Autodesk Inventor part; units mm, degrees
ref_plane "YZ Plane" through (0, 0, 0) normal (1, 0, 0) x (0, 1, 0)
ref_plane "XZ Plane" through (0, 0, 0) normal (0, 1, 0) x (-1, 0, 0)
ref_plane "XY Plane" through (0, 0, 0) normal (0, 0, 1) x (1, 0, 0)
sketch "Boceto1" plane through (0, 0, 0) normal (0, 1, 0) x (-1, 0, 0)
  line L0 (0, 0) -> (11, 0)
  line L1 (11, 0) -> (11, -11)
  line L2 (11, -11) -> (0, -11)
  line L3 (0, -11) -> (0, 0)
  dimension "d0" = 11
  dimension "d1" = 11
extrude "Extrusión1" add sketch "Boceto1" along normal blind 1.25
sketch "Boceto2" plane through (0, 1.25, 0) normal (0, 1, 0) x (1, 0, 0)
  line L0 (-11, 0) -> (0, 0)
  line L1 (-11, 11) -> (-11, 0)
  line L2 (0, 0) -> (-11, 11)
  line L3 (0, 0) -> (0, 11)
  line L4 (0, 11) -> (-11, 0)
  circle A0 centre (-5.5, 5.5) radius 5.5
  dimension "d4" = 11
extrude "Extrusión2" add sketch "Boceto2" along normal blind 6 contours A0 L4 L2 | A0 L2 L4 | L2 L4 A0 | A0 L4 L2
sketch "Boceto4" plane through (-5.5, 7.25, -5.5) normal (0, 1, 0) x (1, 0, 0)
  line L0 (0, 0) -> (-3, 0)
  line L1 (-3, 0) -> (-3, 1.5)
  line L2 (-3, 1.5) -> (-3, -1.5)
  line L3 (-3, -1.5) -> (-1.5, -1.5)
  line L4 (-1.5, -1.5) -> (-1.5, -3)
  line L5 (-1.5, -3) -> (1.5, -3)
  line L6 (1.5, -3) -> (1.5, -1.5)
  line L7 (1.5, -1.5) -> (3, -1.5)
  line L8 (3, -1.5) -> (3, 1.5)
  line L9 (3, 1.5) -> (1.5, 1.5)
  line L10 (1.5, 1.5) -> (1.5, 3)
  line L11 (1.5, 3) -> (-1.5, 3)
  line L12 (-1.5, 3) -> (-1.5, 1.5)
  line L13 (-3, 1.5) -> (-1.5, 1.5)
  line L14 (-1.5, 1.5) -> (-1.5, -1.5)
  line L15 (1.5, -1.5) -> (1.5, 1.5)
  line L16 (-1.5, 1.5) -> (1.5, 1.5)
  line L17 (1.5, -1.5) -> (-1.5, -1.5)
  point P0 (5.5, -5.5)
  dimension "d7" = 3
  dimension "d8" = 1.5
  dimension "d9" = 3
  dimension "d10" = 1.5
  dimension "d11" = 1.5
  dimension "d12" = 3
  dimension "d13" = 1.5
  dimension "d14" = 1.5
  dimension "d15" = 3
  dimension "d16" = 1.5
  dimension "d17" = 1.5
  dimension "d18" = 3
extrude "Extrusión3" cut sketch "Boceto4" against normal blind 5 contours L14 L16 L15 L17
sketch "Boceto8" plane through (-5.5, 7.25, -5.5) normal (0, 1, 0) x (1, 0, 0)
  circle A0 centre (0, 0) radius 2.75
  circle A1 centre (0, 0) radius 4.5
  point P0 (5.5, -5.5)
  dimension "d47" = 5.5
  dimension "d48" = 9
extrude "Extrusión6" cut sketch "Boceto8" against normal blind 2
fillet "Empalme4" radius 1 4 edges at (-7, 4.75, -7) (-4, 4.75, -7) (-4, 4.75, -4) (-7, 4.75, -4)
properties part number "Boton Base"
Verification items for the finished model (mm, model axes). A direction names the side the tool comes from. Round coordinates to 2 decimals unless told otherwise and drop trailing zeros. Order: outer loops, then holes, each group sorted by start corner. A loop starts at its lowest first (then second) coordinate and runs counter-clockwise, first axis right, second up. Notation, with made-up numbers: (40.5, 73.5) -> (95.5, 73.5) arc R27 ccw to (95.5, 103.5) -> close; hole circle Ø11 at (29.25, 76). An arc over 180 degrees is marked (long way). Put each result on its own line as item: value. Start each with the question number.
(1) Section check B-B (y = 3.5). Enter the section's corners in (x, z), then the cut area to 3 significant figures.
(2) Tool access check on faces 5 (the face through (-10, 1.25, -10)), 6 (the face through (-4.301, 4.715, -6.715)), 7 (the face through (-10, 1.25, -1)). Record the directions out of +Z, -Z, +X, -X, +Y, -Y that give a thin tool (end or side, any length) a straight path to the whole face; none if there is none.
(3) Section check D-D (x = -2.25). Enter the section's corners in (y, z), then the cut area to 3 significant figures.
(4) Section check A-A (y = 6). Enter the section's corners in (x, z).
(5) Depth check by flat-ended pin: pin 1 Ø2 at (x, y) = (-4.5, 4) entering from -Z; pin 2 Ø3 at (x, y) = (-2.5, 6.5) entering from -Z; pin 3 Ø1 at (y, z) = (3.5, -1.5) entering from -X. Enter the tip coordinate at first touch or a pass-through.
(6) Draft check along Z on faces 1 (the face through (0, 1, -6)), 2 (the face through (-6, 1, -11)), 3 (the face through (-6.69, 4.21, -10.87)), 4 (the face through (-4.23, 6.26, -3.06)). Enter one of: +Z half, -Z half, draft (parallel to the pull), parting line (faces both ways), or undercut.
(7) Material ranges on line 1 along X through (y, z) = (6.8, -5.5); line 2 along Z through (x, y) = (-6.25, 6.75), recorded low to high.
(8) Section check C-C (z = -9.75). Enter the section's corners in (x, y).
Completed:
1. outline: circle Ø11 at (-5.5, -5.5); hole (-7, -6) arc R1 ccw to (-6, -7) -> (-5, -7) arc R1 ccw to (-4, -6) -> (-4, -5) arc R1 ccw to (-5, -4) -> (-6, -4) arc R1 ccw to (-7, -5) -> close
1. area: 86.9 mm2
2. face 5: -Z, -X, +Y
2. face 6: +Y
2. face 7: +Z, -X, +Y
3. outline: (0, -11) -> (1.25, -11) -> (1.25, -9.94) -> (7.25, -9.94) -> (7.25, -8.61) -> (5.25, -8.61) -> (5.25, -2.39) -> (7.25, -2.39) -> (7.25, -1.06) -> (1.25, -1.06) -> (1.25, 0) -> (0, 0) -> close
3. area: 54.5 mm2
4. outline: circle Ø11 at (-5.5, -5.5); circle Ø5.5 at (-5.5, -5.5); hole circle Ø9 at (-5.5, -5.5); hole (-7, -6) arc R1 ccw to (-6, -7) -> (-5, -7) arc R1 ccw to (-4, -6) -> (-4, -5) arc R1 ccw to (-5, -4) -> (-6, -4) arc R1 ccw to (-7, -5) -> close
5. pin 1: stops at z = -11
5. pin 2: stops at z = -10.79
5. pin 3: stops at x = -9.74
6. face 1: draft
6. face 2: -Z half
6. face 3: parting line
6. face 4: undercut
7. line 1: x = -11 to -10, -8.25 to -7, -4 to -2.75, -1 to 0
7. line 2: z = -10.95 to -9.94, -8.15 to -6.97, -4.03 to -2.85, -1.06 to -0.05
8. outline: (-11, 0) -> (0, 0) -> (0, 1.25) -> (-2.01, 1.25) -> (-2.01, 7.25) -> (-4.02, 7.25) -> (-4.02, 5.25) -> (-6.98, 5.25) -> (-6.98, 7.25) -> (-8.99, 7.25) -> (-8.99, 1.25) -> (-11, 1.25) -> close
